from build123d import *

# Parameters (mm, degrees)
F1_DEPTH     = 19.05
F2_DEPTH     = 114.3
F3_W         = 114.3
F3_H         = 101.6
F4_DEPTH     = 177.8
F5_T1_DEPTH  = 641.9538230647
F6_R         = 37.1475
F7_DEPTH     = 25.4
F8_R         = 37.1475
F9_DEPTH     = 25.4
F10_W        = 114.3
F10_H        = 266.7
F11_DEPTH    = 38.1
F12_T4_DEPTH = 574.9754388191
F13_T1_DEPTH = 442.85989084
F14_START    = 88.9
F14_DEPTH    = 25.4


# Not quite as in the source:
# - a fillet or chamfer that OpenCascade refuses, or shapes differently, is made with other operations: its cross-section is extruded or revolved along the edge and cut away or added


with BuildPart() as f1:
    # F0 (on Right) → F1 (new body)
    with BuildSketch(Plane.YZ):
        with BuildLine():
            Line((50.8, -101.6), (50.8, 0))
            ThreePointArc((50.8, 0), (0, -50.8), (-50.8, 0))
            Line((-50.8, 0), (-50.8, -101.6))
            Line((-50.8, -101.6), (50.8, -101.6))
        make_face()
    extrude(amount=F1_DEPTH)

    # F0 (on Right) → F2 (join)
    with BuildSketch(Plane.YZ):
        with BuildLine():
            Line((50.8, -101.6), (50.8, 0))
            ThreePointArc((50.8, 0), (0, -50.8), (-50.8, 0))
            Line((-50.8, 0), (-50.8, -101.6))
            Line((-50.8, -101.6), (50.8, -101.6))
        make_face()
    extrude(amount=F2_DEPTH)

    # F3 (on face) → F4 (join)
    with BuildSketch(Plane(origin=(0, 0, -101.6), x_dir=(1, 0, 0), z_dir=(0, 0, -1))):
        with Locations((57.15, 0)):
            Rectangle(F3_W, F3_H)
    extrude(amount=F4_DEPTH)

    # F5: chamfer of 101.6 x 27.223637951 on 1 edges, made by hand

    # F5_s2 → F5_t1 (cut)
    with BuildSketch(Plane.YZ.offset(-263.8269115324)):
        Polygon((23.576362049, -279.4), (50.8, -177.8), (50.8, -279.4), align=None)
    extrude(amount=F5_T1_DEPTH, mode=Mode.SUBTRACT)

    # F6 (on face) → F7 (join)
    with BuildSketch(Plane(origin=(0, 0, 0), x_dir=(0, -1, 0), z_dir=(-1, 0, 0))):
        with Locations((13.6118189755, -279.4)):
            Circle(F6_R)
    extrude(amount=-F7_DEPTH)

    # F8 (on face) → F9 (join)
    with BuildSketch(Plane.YZ.offset(114.3)):
        with Locations((-13.6118189755, -279.4)):
            Circle(F8_R)
    extrude(amount=-F9_DEPTH)

    # F10 (on face) → F11 (join)
    with BuildSketch(Plane.XZ.offset(50.8)):
        with Locations((57.15, -133.35)):
            Rectangle(F10_W, F10_H)
    extrude(amount=F11_DEPTH)

    # F12: chamfer of 88.9 x 41.45475081 on 1 edges, made by hand


with BuildPart() as f12_tool2:
    # F12_s3 → F12_t4 (new body)
    with BuildSketch(Plane.YZ.offset(-230.3377194096)):
        Polygon((-88.9, -177.8), (-47.44524919, -266.7), (-88.9, -266.7), align=None)
    extrude(amount=F12_T4_DEPTH)

    split(bisect_by=Plane.XZ.offset(50.8), keep=Keep.TOP)


with BuildPart() as f1_1:
    add(f1.part)

    # F12_t1: cut F12_tool2
    add(f12_tool2.part, mode=Mode.SUBTRACT)

    # F13: chamfer of 63.5 x 36.6617420935 on 1 edges, made by hand

    # F13_s2 → F13_t1 (cut)
    with BuildSketch(Plane.YZ.offset(-164.27994542)):
        Polygon((-88.9, -63.5), (-52.2382579065, 0), (-88.9, 0), align=None)
    extrude(amount=F13_T1_DEPTH, mode=Mode.SUBTRACT)

    # F0 (on Right) → F14 (join)
    with BuildSketch(Plane.YZ.offset(F14_START)):
        with BuildLine():
            Line((-50.8, 0), (50.8, 0))
            ThreePointArc((50.8, 0), (0, 50.8), (-50.8, 0))
        make_face()
        with BuildLine():
            ThreePointArc((-50.8, 0), (0, -50.8), (50.8, 0))
            Line((50.8, 0), (-50.8, 0))
        make_face()
    extrude(amount=F14_DEPTH)


solid = f1_1.part
Geometry check sheet. Reference: the model listing, model coordinates, mm. A direction names the side the tool comes from. Give positions to 0.01 mm unless a question says otherwise; leave off trailing zeros. Loops run counter-clockwise (first coordinate to the right, second up) from the corner with the lowest first, then second, coordinate; pieces in that order, holes last. Notation, with made-up numbers: (14, -5.75) -> (28, -5.75) arc R33 ccw to (28, 33.25) -> close; hole circle Ø3 at (-13.75, 37). An arc over 180 degrees is marked (long way). Answer in a Markdown table with one row per item. Add a question column.
1) Cross-section at A-A on z = -293. Record the boundary of the cut face in (x, y).
2) Cross-section at D-D on x = 82. Record the boundary of the cut face in (y, z), and give its area (3 significant figures).
3) Draft check along X on faces 4 (the face through (25.4, -13, -294)), 5 (the face through (114.3, -20, -130)), 6 (the face through (101.78, -14.43, -316.54)), 7 (the face through (88.9, -1, 1)). Enter one of: pulls with the +X half, pulls with the -X half, needs draft (parallel to the pull), parting line crosses it, or undercut.
4) Gauge pin test, flat ends, axial feed: P1, Ø16, axis at x = 47, z = -272.5, coming from the -Y side; P2, Ø8, axis at x = 67.5, y = -17.5, coming from the +Z side; P3, Ø1, axis at x = 24.5, z = -18, coming from the -Y side. Record the tip position at first contact, or that the pin passes through.
5) Cross-section at C-C on y = -5. Record the boundary of the cut face in (x, z), and give its area (3 significant figures).
6) Set-up check for faces 1 (the face through (56, -50.8, -269)), 2 (the face through (43.828, 1.117, -50.788)), 3 (the face through (88.9, -14, -294)): record each of +Z, -Z, +X, -X, +Y, -Y from which the full face is reachable in a straight line by a thin tool's end or side.
7) Material ranges on probe 1 along X at (y, z) = (10.5, -296.5); probe 2 along X at (y, z) = (-38, 8.5); probe 3 along Y at (x, z) = (13, -14), recorded low to high. Write a range as from..to.
Outcome:
| question | item | result |
|---|---|---|
| 1 | outline | (0, -48.18) -> (25.4, -48.18) -> (25.4, 20.96) -> (0, 20.96) -> close; (88.9, -48.18) -> (114.3, -48.18) -> (114.3, 20.96) -> (88.9, 20.96) -> close |
| 2 | outline | (-88.9, -177.8) -> (-50.8, -259.51) -> (-50.8, -279.4) -> (23.58, -279.4) -> (50.8, -177.8) -> (50.8, 0) arc R50.8 cw to (-50.8, 0) -> (-52.24, 0) -> (-88.9, -63.5) -> close |
| 2 | area | 30,100 mm^2 |
| 3 | face 4 | undercut |
| 3 | face 5 | pulls with the +X half |
| 3 | face 6 | needs draft |
| 3 | face 7 | pulls with the -X half |
| 4 | P1 | stops at y = -50.8 |
| 4 | P2 | stops at z = -46.03 |
| 4 | P3 | stops at y = -62.92 |
| 5 | outline | (0, -315.54) -> (25.4, -315.54) -> (25.4, -279.4) -> (88.9, -279.4) -> (88.9, -315.54) -> (114.3, -315.54) -> (114.3, 50.55) -> (88.9, 50.55) -> (88.9, -50.55) -> (0, -50.55) -> close |
| 5 | area | 30,600 mm^2 |
| 6 | face 1 | -Z, +X, -X, -Y |
| 6 | face 2 | +Z, -X |
| 6 | face 3 | -Z, +Y, -Y |
| 7 | probe 1 | x = 0..25.4, 88.9..114.3 |
| 7 | probe 2 | x = 88.9..114.3 |
| 7 | probe 3 | y = -60.32..-48.83, 48.83..50.8 |
